Here's how the part is built. I have some questions about the finished solid (model axes, mm). Face numbers are marked on the shaded views. Round coordinates to 2 decimals unless told otherwise and drop trailing zeros. Order: outer loops, then holes, each group sorted by start corner. A loop starts at its lowest first (then second) coordinate and runs counter-clockwise, first axis right, second up. Notation, with made-up numbers: (-16.75, -15) -> (29.25, -15) arc R26 cw to (29.25, 4) -> close; hole circle Ø1 at (74.5, 28.5). An arc over 180 degrees is marked (long way). Answer in a Markdown table with one row per item.
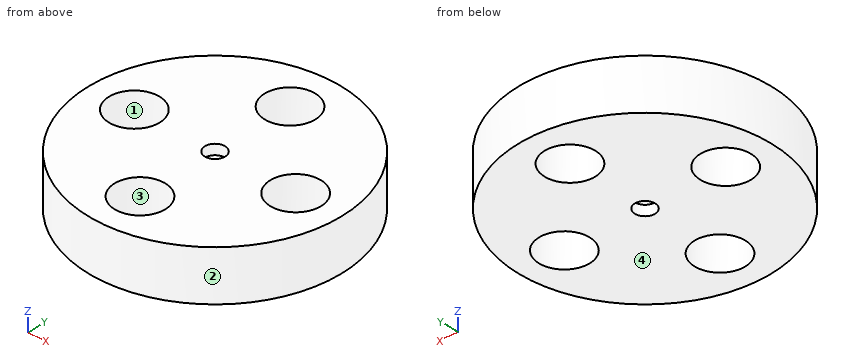
```python
from build123d import *

# Parameters (mm, degrees)
F0_R     = 12.5
F0_R_2   = 2.5
F1_DEPTH = 5
F2_R     = 1
F3_DEPTH = 1
F4_R     = 1
F5_DEPTH = 1


with BuildPart() as f1:
    # F0 (on Top) → F1 (new body)
    with BuildSketch(Plane.XY):
        Circle(F0_R)
        with Locations((0, -8)):
            Circle(F0_R_2, mode=Mode.SUBTRACT)
        with Locations((-8, 0)):
            Circle(F0_R_2, mode=Mode.SUBTRACT)
        with Locations((8, 0)):
            Circle(F0_R_2, mode=Mode.SUBTRACT)
        with Locations((0, 8)):
            Circle(F0_R_2, mode=Mode.SUBTRACT)
    extrude(amount=F1_DEPTH)

    # F2 (on face) → F3 (cut)
    with BuildSketch(Plane.XY.offset(5)):
        Circle(F2_R)
    extrude(amount=-F3_DEPTH, mode=Mode.SUBTRACT)

    # F4 (on face) → F5 (cut)
    with BuildSketch(Plane(origin=(0, 0, 0), x_dir=(1, 0, 0), z_dir=(0, 0, -1))):
        Circle(F4_R)
    extrude(amount=-F5_DEPTH, mode=Mode.SUBTRACT)


solid = f1.part
```
1. Suppose I cut it at C-C on x = -2. Write out the boundary of the cut face in (y, z).
Numbers:
| item | result |
|---|---|
| outline | (-12.34, 0) -> (-9.5, 0) -> (-9.5, 5) -> (-12.34, 5) -> close; (-6.5, 0) -> (6.5, 0) -> (6.5, 5) -> (-6.5, 5) -> close; (9.5, 0) -> (12.34, 0) -> (12.34, 5) -> (9.5, 5) -> close |
2. Suppose I cut it at A-A on y = 0. Write out the boundary of the cut face in (x, z).
Numbers:
| item | result |
|---|---|
| outline | (-12.5, 0) -> (-10.5, 0) -> (-10.5, 5) -> (-12.5, 5) -> close; (-5.5, 0) -> (-1, 0) -> (-1, 1) -> (1, 1) -> (1, 0) -> (5.5, 0) -> (5.5, 5) -> (1, 5) -> (1, 4) -> (-1, 4) -> (-1, 5) -> (-5.5, 5) -> close; (10.5, 0) -> (12.5, 0) -> (12.5, 5) -> (10.5, 5) -> close |
3. We'd pull the mould along X, two halves only. Please class the marked faces 1, 2, 3 and 4: released by +X, released by -X, zero draft, split by the parting line, or undercut.
Numbers:
| item | result |
|---|---|
| face 1 | undercut |
| face 2 | split by the parting line |
| face 3 | undercut |
| face 4 | zero draft |
4. Please list where these lines run through material, in increasing order: line 1 along Y through (x, z) = (0, 0.65); line 2 along Y through (x, z) = (0, 1.5); line 3 along X through (y, z) = (0.25, 1.1).
Numbers:
| item | result |
|---|---|
| line 1 | y = -12.5 to -10.5, -5.5 to -1, 1 to 5.5, 10.5 to 12.5 |
| line 2 | y = -12.5 to -10.5, -5.5 to 5.5, 10.5 to 12.5 |
| line 3 | x = -12.5 to -10.49, -5.51 to 5.51, 10.49 to 12.5 |
5. Suppose I cut it at D-D on x = 8. Write out the boundary of the cut face in (y, z).
Numbers:
| item | result |
|---|---|
| outline | (-9.6, 0) -> (-2.5, 0) -> (-2.5, 5) -> (-9.6, 5) -> close; (2.5, 0) -> (9.6, 0) -> (9.6, 5) -> (2.5, 5) -> close |
6. For pin 1 Ø8 at (x, y) = (0, 8) entering from -Z; pin 2 Ø1.8 at (x, y) = (0, 0) entering from -Z; pin 3 Ø0.6 at (x, y) = (0, 0) entering from +Z, each with a flat end and sliding along its axis, tell me the tip position at first contact or that it passes through.
Numbers:
| item | result |
|---|---|
| pin 1 | stops at z = 0 |
| pin 2 | stops at z = 1 |
| pin 3 | stops at z = 4 |
7. Suppose I cut it at B-B on z = 4.6. Write out the boundary of the cut face in (x, y).
Numbers:
| item | result |
|---|---|
| outline | circle Ø25 at (0, 0); hole circle Ø5 at (-8, 0); hole circle Ø5 at (0, -8); hole circle Ø5 at (0, 8); hole circle Ø2 at (0, 0); hole circle Ø5 at (8, 0) |
